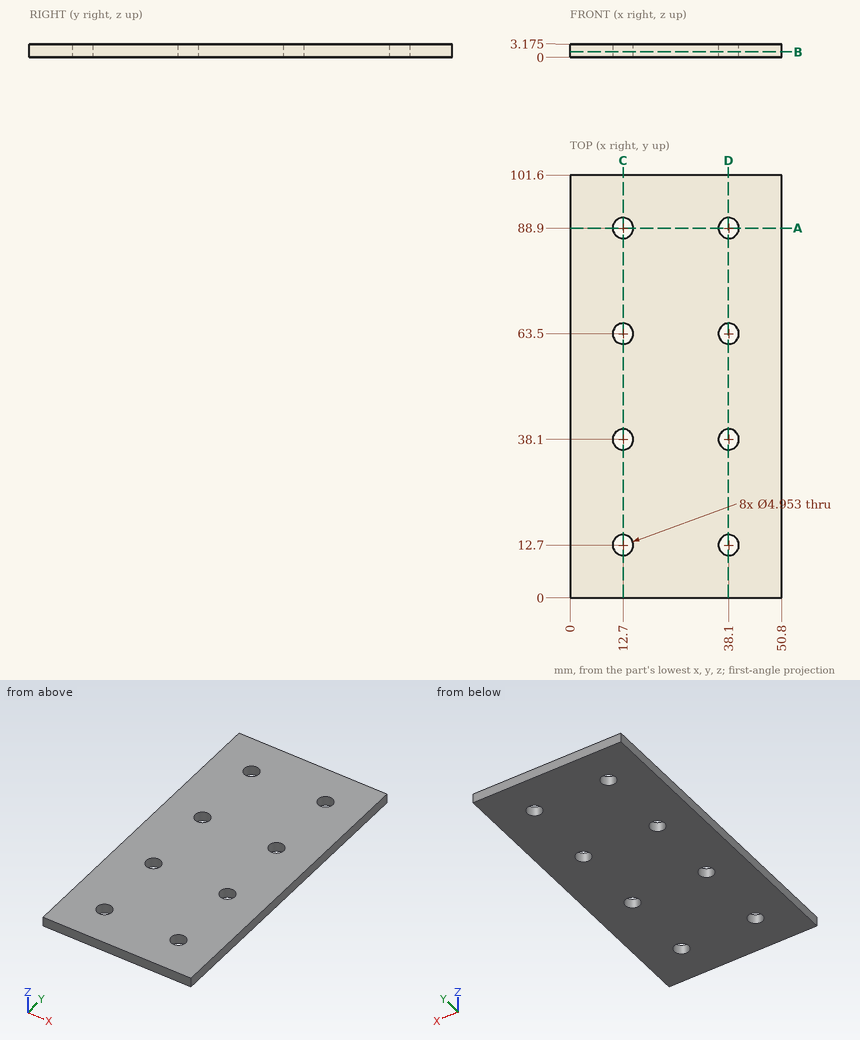
The figure shows three views and two pictorial views of one solid part (mm, origin at its lowest corner). Answer the questions. Give positions to 0.01 mm unless a question says otherwise; leave off trailing zeros. Write each loop counter-clockwise with the first axis right and the second up, starting at its lowest first coordinate (ties: lowest second). Pieces come first, ordered by that corner, then holes. Notation, with made-up numbers: (45.5, 31) -> (80.5, 31) arc R17 cw to (80.5, 62) -> close; hole circle Ø5 at (55.5, 41.5). An arc over 180 degrees is marked (long way). Write each question's results on one line, items separated by ' | '.
1. Find section C-C on x = 12.7. Determine the outline of the cut face in (y, z) (1 decimal).
Data:
outline: (0, 0) -> (10.2, 0) -> (10.2, 3.2) -> (0, 3.2) -> close; (15.2, 0) -> (35.6, 0) -> (35.6, 3.2) -> (15.2, 3.2) -> close; (40.6, 0) -> (61, 0) -> (61, 3.2) -> (40.6, 3.2) -> close; (66, 0) -> (86.4, 0) -> (86.4, 3.2) -> (66, 3.2) -> close; (91.4, 0) -> (101.6, 0) -> (101.6, 3.2) -> (91.4, 3.2) -> close
2. Straight lines are drawn through the part: L1, parallel to Y at x = 38.1, z = 1.05; L2, parallel to X at y = 89, z = 2.6; L3, parallel to X at y = 65.5, z = 2.1. For each, find the intervals that lie inside material, in ascending order.
Data:
L1: 0 to 10.22, 15.18 to 35.62, 40.58 to 61.02, 65.98 to 86.42, 91.38 to 101.6 | L2: 0 to 10.23, 15.17 to 35.63, 40.57 to 50.8 | L3: 0 to 11.24, 14.16 to 36.64, 39.56 to 50.8
3. Find section A-A on y = 88.9. Determine the outline of the cut face in (x, z) (1 decimal).
Data:
outline: (0, 0) -> (10.2, 0) -> (10.2, 3.2) -> (0, 3.2) -> close; (15.2, 0) -> (35.6, 0) -> (35.6, 3.2) -> (15.2, 3.2) -> close; (40.6, 0) -> (50.8, 0) -> (50.8, 3.2) -> (40.6, 3.2) -> close
4. Find section D-D on x = 38. Determine the outline of the cut face in (y, z) (3 decimals).
Data:
outline: (0, 0) -> (10.226, 0) -> (10.226, 3.175) -> (0, 3.175) -> close; (15.174, 0) -> (35.626, 0) -> (35.626, 3.175) -> (15.174, 3.175) -> close; (40.574, 0) -> (61.026, 0) -> (61.026, 3.175) -> (40.574, 3.175) -> close; (65.974, 0) -> (86.426, 0) -> (86.426, 3.175) -> (65.974, 3.175) -> close; (91.374, 0) -> (101.6, 0) -> (101.6, 3.175) -> (91.374, 3.175) -> close
5. Find section B-B on z = 1.3. Give the number of separate pieces and of enclosed holes in the cut face, and give its area (3 significant figures).
Data:
separate pieces: 1 | enclosed holes: 8 | area: 5,010 mm^2
6. This flat-tipped pin is pushed along its axis until it touches: pin 1 Ø3 at (x, y) = (12.7, 38.1) entering from -Z. Where does it stop, or does it pass through?
Data:
pin 1: through
